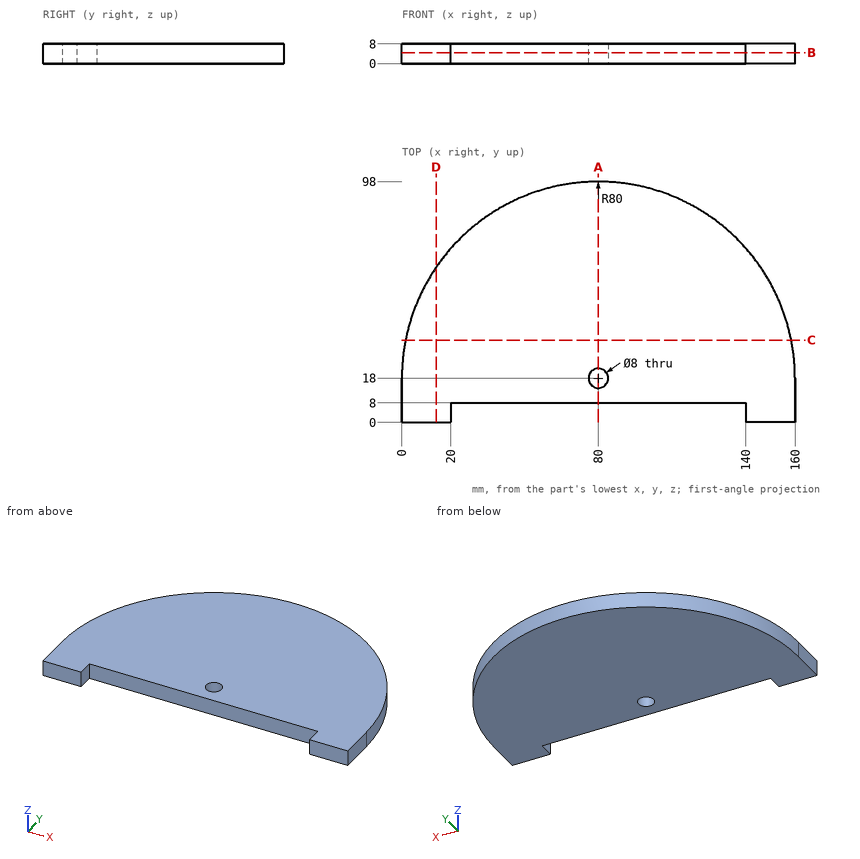
Design review of the part shown in the three views and the two pictorial views. Dimensions are in mm from the part's minimum x, y and z. Give positions to 0.01 mm unless a question says otherwise; leave off trailing zeros. Loops run counter-clockwise (first coordinate to the right, second up) from the corner with the lowest first, then second, coordinate; pieces in that order, holes last. Notation, with made-up numbers: (20.5, 57) -> (36.5, 57) arc R15 ccw to (36.5, 62) -> close; hole circle Ø2 at (12, 89). An arc over 180 degrees is marked (long way). One line per question, with ' | ' between items.
1) To check wall thickness, follow probe 1 along Y at (x, z) = (80, 5.25); probe 2 along X at (y, z) = (7.5, 3.25); probe 3 along X at (y, z) = (18.5, 7.5). State the ranges of each line that lie inside material, in increasing order.
Resolved:
probe 1: y = 8 to 14, 22 to 98 | probe 2: x = 0 to 20, 140 to 160 | probe 3: x = 0 to 76.03, 83.97 to 160
2) We need section B-B (z = 4.5). Write out the cut boundary in (x, y), plus the area to 3 significant figures.
Resolved:
outline: (0, 0) -> (20, 0) -> (20, 8) -> (140, 8) -> (140, 0) -> (160, 0) -> (160, 18) arc R80 ccw to (0, 18) -> close; hole circle Ø8 at (80, 18) | area: 11,900 mm2
3) We need section D-D (x = 14). Write out the cut boundary in (y, z), plus the area to 3 significant figures.
Resolved:
outline: (0, 0) -> (63.21, 0) -> (63.21, 8) -> (0, 8) -> close | area: 506 mm2
4) We need section C-C (y = 33.5). Write out the cut boundary in (x, z).
Resolved:
outline: (1.52, 0) -> (158.48, 0) -> (158.48, 8) -> (1.52, 8) -> close
5) We need section A-A (x = 80). Write out the cut boundary in (y, z).
Resolved:
outline: (8, 0) -> (14, 0) -> (14, 8) -> (8, 8) -> close; (22, 0) -> (98, 0) -> (98, 8) -> (22, 8) -> close
6) Insertion check: pin 1 Ø3 at (x, z) = (24.5, 3) entering from +Y; pin 2 Ø2.5 at (x, z) = (97.5, 2) entering from -Y. Each pin has a flat end and moves straight along its axis. Give the tip position at first contact, or say it passes through.
Resolved:
pin 1: stops at y = 77.03 | pin 2: stops at y = 8
